Could you check a few things on this model? Use its own coordinates, in mm. A direction names the side the tool comes from. Coordinates: 2 decimals unless noted, no trailing zeros. Write each loop counter-clockwise with the first axis right and the second up, starting at its lowest first coordinate (ties: lowest second). Pieces come first, ordered by that corner, then holes.
Item 1: For P1, Ø1.6, axis at x = -0.5, z = 0.5, coming from the -Y side; P2, Ø1.8, axis at x = 0, z = 0, coming from the -Y side (3 decimals), each with a flat end and sliding along its axis, tell me the tip position at first contact or that it passes through.
Item 2: If I drill on probe 1 along Z at (x, y) = (0, 2.1); probe 2 along Y at (x, z) = (-3.75, 3.75) (3 decimals); probe 3 along X at (y, z) = (2.25, -3.75), over which ranges is the centre line in solid material (lowest first)?
Item 3: Which directions (+Z, -Z, +X, -X, +Y, -Y) give clear straight access to the entire face, cutting with the end or side of a thin tool? Please do faces 4 (the flat face through (-0.1, 0, -1.2)), 5 (the flat face through (0, 3.175, 0)).
Item 4: I want a section at C-C on z = 0. Please give me the cut outline in (x, y) (3 decimals).
Item 5: Thinking about a two-plate mould opening in X: for faces 1 (the flat face through (-2, 3.175, -5)), 2 (the flat face through (-7.5, 4, 0)), 3 (the cylindrical face through (0, 2, -1)), which applies, +X half, -X half, draft (parallel to the pull), parting line (faces both ways), or undercut?
Item 6: I want a section at D-D on z = 6.25. Please give me the cut outline in (x, y) (3 decimals), then the cut area to 3 significant figures.
Item 7: I want a section at B-B on y = 2.9. Please give me the cut outline in (x, z).
Item 8: I want a section at A-A on x = 0. Please give me the cut outline in (y, z) (3 decimals), then the cut area to 3 significant figures.
from build123d import *

# Parameters (mm, degrees)
SKETCH1_R           = 5
BOSS_EXTRUDE1_DEPTH = 3.175
SKETCH2_R           = 1
CUT_EXTRUDE1_DEPTH  = 3.175
SKETCH3_W           = 15
SKETCH3_H           = 15
BOSS_EXTRUDE2_DEPTH = 2


with BuildPart() as part:
    # Sketch1 → Boss-Extrude1 (new body)
    with BuildSketch(Plane(origin=(0, 0, 0), x_dir=(1, 0, 0), z_dir=(0, 1, 0))):
        Circle(SKETCH1_R)
    extrude(amount=BOSS_EXTRUDE1_DEPTH)

    # Sketch2 → Cut-Extrude1 (cut)
    with BuildSketch(Plane.XZ):
        Circle(SKETCH2_R)
    extrude(amount=-CUT_EXTRUDE1_DEPTH, mode=Mode.SUBTRACT)

    # Sketch3 → Boss-Extrude2 (add)
    with BuildSketch(Plane(origin=(0, 3.175, 0), x_dir=(1, 0, 0), z_dir=(0, 1, 0))):
        Rectangle(SKETCH3_W, SKETCH3_H)
    extrude(amount=BOSS_EXTRUDE2_DEPTH)


solid = part.part
Response values:
1. P1: stops at y = 0
1. P2: stops at y = 3.175
2. probe 1: z = -5 to -1, 1 to 5
2. probe 2: y = 3.175 to 5.175
2. probe 3: x = -3.31 to 3.31
3. face 4: +Z, -Z, +X, -X, -Y
3. face 5: -Y
4. outline: (-7.5, 3.175) - (-5, 3.175) - (-5, 0) - (-1, 0) - (-1, 3.175) - (1, 3.175) - (1, 0) - (5, 0) - (5, 3.175) - (7.5, 3.175) - (7.5, 5.175) - (-7.5, 5.175) - close
5. face 1: draft
5. face 2: -X half
5. face 3: undercut
6. outline: (-7.5, 3.175) - (7.5, 3.175) - (7.5, 5.175) - (-7.5, 5.175) - close
6. area: 30.0 mm2
7. outline: circle Ø10 at (0, 0); hole circle Ø2 at (0, 0)
8. outline: (0, -5) - (3.175, -5) - (3.175, -7.5) - (5.175, -7.5) - (5.175, 7.5) - (3.175, 7.5) - (3.175, 5) - (0, 5) - (0, 1) - (3.175, 1) - (3.175, -1) - (0, -1) - close
8. area: 55.4 mm2
